Design review of the part built by this model. Coordinates are the model's own, in mm. Face numbers are marked on the shaded views. Coordinates: 2 decimals unless noted, no trailing zeros. Loops run counter-clockwise (first coordinate to the right, second up) from the corner with the lowest first, then second, coordinate; pieces in that order, holes last. Notation, with made-up numbers: (-14, 29) -> (-1, 29) arc R33 ccw to (-1, 66) -> close; hole circle Ø5 at (-17.75, -35). An arc over 180 degrees is marked (long way). Use a Markdown table: item, result. Add a question column.
Q1. Take a section at A-A on x = 0. Write out the cut boundary in (y, z), plus the area to 3 significant figures.
Q2. Take a section at D-D on z = -1.75. Write out the cut boundary in (x, y), plus the area to 3 significant figures.
Q3. For probe 1 along Y at (x, z) = (0, 0.3); probe 2 along Y at (x, z) = (0, 1.55); probe 3 along Y at (x, z) = (-7.5, 1.25), list the stretches that pass through material, from the lowest coordinate up.
Q4. Clearance check with flat-ended pins moving along their axes: pin 1 Ø1 at (x, z) = (0.5, -5) entering from +Y; pin 2 Ø1 at (x, y) = (7, -6) entering from -Z; pin 3 Ø5 at (y, z) = (-0.5, 5) entering from +X; pin 4 Ø1 at (y, z) = (0, 5) entering from +X. State where each tip first meets the part, or that it passes through.
Q5. Take a section at C-C on z = 1.25. Write out the cut boundary in (x, y).
Q6. Draft analysis for pull direction X (two halves, no side actions). For the marked faces 1 and 2, state which applies: pulls with the +X half, pulls with the -X half, needs draft (parallel to the pull), parting line crosses it, or undercut.
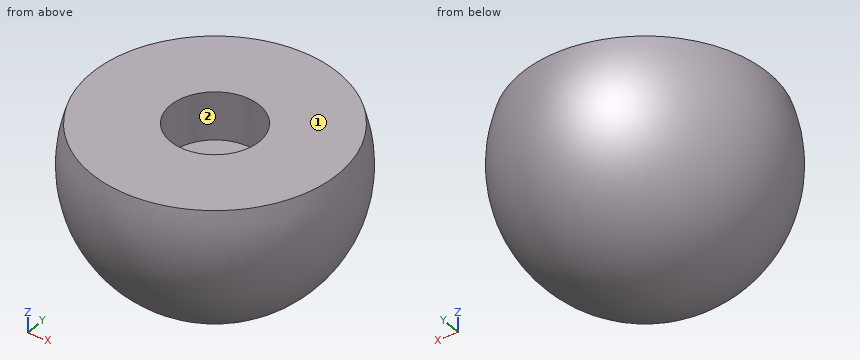
from build123d import *

# Parameters (mm, degrees)
F2_W     = 25.694864
F2_H     = 24.584594
F3_DEPTH = 25
F6_R     = 3.25
F7_DEPTH = 3.5


with BuildPart() as f1:
    # F0 (on Right) → F1 (revolve)
    with BuildSketch(Plane.YZ):
        with BuildLine():
            Line((9.5, 0), (-9.5, 0))
            ThreePointArc((-9.5, 0), (0, -9.5), (9.5, 0))
        make_face()
    revolve(axis=Axis((0, 0, 0), (0, 1, 0)))


with BuildPart() as f3:
    # F2 (on Top) → F3 (new body)
    with BuildSketch(Plane.XY):
        Rectangle(F2_W, F2_H)
    extrude(amount=F3_DEPTH)


with BuildPart() as f3_1:
    # F4: moved
    add(f3.part.moved(Location((0, 0, 3))))


with BuildPart() as f1_1:
    add(f1.part)

    # F5: cut F3
    add(f3_1.part, mode=Mode.SUBTRACT)

    # F6 (on face) → F7 (cut)
    with BuildSketch(Plane.XY.offset(3)):
        Circle(F6_R)
    extrude(amount=-F7_DEPTH, mode=Mode.SUBTRACT)


solid = f1_1.part
Answer list:
| question | item | result |
|---|---|---|
| 1 | outline | (-9.01, 3) arc R9.5 ccw (long way) to (9.01, 3) -> (3.25, 3) -> (3.25, -0.5) -> (-3.25, -0.5) -> (-3.25, 3) -> close |
| 1 | area | 175 mm² |
| 2 | outline | circle Ø18.67 at (0, 0) |
| 2 | area | 274 mm² |
| 3 | probe 1 | -9.5 to -3.25, 3.25 to 9.5 |
| 3 | probe 2 | -9.37 to -3.25, 3.25 to 9.37 |
| 3 | probe 3 | -5.7 to 5.7 |
| 4 | pin 1 | y = 8.35 |
| 4 | pin 2 | z = -3.77 |
| 4 | pin 3 | x = 9.16 |
| 4 | pin 4 | through |
| 5 | outline | circle Ø18.83 at (0, 0); hole circle Ø6.5 at (0, 0) |
| 6 | face 1 | needs draft |
| 6 | face 2 | undercut |
